```python
from build123d import *

# Parameters (mm, degrees)
F2_DEPTH    = 11.43
F0_W        = 4.9775806256
F0_H        = 21.5646
F3_DEPTH    = 3.556
F4_T1_DEPTH = 27.2262824301


# Not quite as in the source:
# - a fillet or chamfer that OpenCascade refuses, or shapes differently, is made with other operations: its cross-section is extruded or revolved along the edge and cut away or added


with BuildPart() as f2:
    # F1 (on Top) → F2 (new body)
    with BuildSketch(Plane.XY):
        with BuildLine():
            ThreePointArc((11.1534688622, 0), (0, 6.4792498177), (-11.1534688622, 0))
            Line((-11.1534688622, 0), (11.1534688622, 0))
        make_face()
    extrude(amount=F2_DEPTH)

    # F0 (on Front) → F3 (join)
    with BuildSketch(Plane.XZ):
        Rectangle(F0_W, F0_H)
    extrude(amount=F3_DEPTH)

    # F4: chamfer of 2.54 on 2 edges, made by hand

    # F4_s2 → F4_t1 (cut)
    with BuildSketch(Plane.XY.offset(-7.898141215)):
        with BuildLine():
            Line((-8.190415898, -0.0933816317), (-9.3391430842, 2.5863339915))
            Line((-9.3391430842, 2.5863339915), (-9.3759354233, 2.6213620343))
            ThreePointArc((-9.3759354233, 2.6213620343), (-10.327366328, 1.3537144774), (-11.1975980412, 0.0251645696))
            Line((-11.1975980412, 0.0251645696), (-11.1534688622, -0.0508))
            ThreePointArc((-11.1534688622, -0.0508), (-9.6719423801, -0.0508), (-8.190415898, -0.1441816317))
            Line((-8.190415898, -0.1441816317), (-8.190415898, -0.0933816317))
        make_face()
        with BuildLine():
            Line((8.190415898, -0.0933816317), (9.3391430842, 2.5863339915))
            Line((9.3391430842, 2.5863339915), (9.3759354233, 2.6213620343))
            ThreePointArc((9.3759354233, 2.6213620343), (10.327366328, 1.3537144774), (11.1975980412, 0.0251645696))
            Line((11.1975980412, 0.0251645696), (11.1534688622, -0.0508))
            ThreePointArc((11.1534688622, -0.0508), (9.6719423801, -0.0508), (8.190415898, -0.1441816317))
            Line((8.190415898, -0.1441816317), (8.190415898, -0.0933816317))
        make_face()
    extrude(amount=F4_T1_DEPTH, mode=Mode.SUBTRACT)


solid = f2.part
```
Verification items for the finished model (mm, model axes). A direction names the side the tool comes from. Coordinates: 2 decimals unless noted, no trailing zeros. Write each loop counter-clockwise with the first axis right and the second up, starting at its lowest first coordinate (ties: lowest second). Pieces come first, ordered by that corner, then holes. Notation, with made-up numbers: M 38.5,72 L 69.5,72 A18 ccw 69.5,103 Z; hole C 38,77 d10. An arc over 180 degrees is marked long. Answer as a JSON object with one key per item and string values. Group by question number.
(1) Gauge pin test, flat ends, axial feed: pin 1 (6 mm diameter, centred on x = 2.5, y = 5.5, fed in from -Z); pin 2 (9 mm diameter, centred on x = -3, z = 8, fed in from -Y); pin 3 (1.1 mm diameter, centred on y = -1, z = 5, fed in from -X); pin 4 (3 mm diameter, centred on y = -2, z = 5.5, fed in from +X). Record the tip position at first contact, or that the pin passes through.
(2) Cross-section at B-B, the plane x = 0. Record the cut outline in (y, z), and give its area (3 significant figures).
(3) Cross-section at C-C, the plane y = -0.5. Record the cut outline in (x, z), and give its area (3 significant figures).
(4) Tool access check on faces 1 (the face through (0, -2, 10.782)), 2 (the face through (2.489, -2, 0)), 3 (the face through (0, 3, 0)), 4 (the face through (-2.489, -2, 0)). Record the directions out of +Z, -Z, +X, -X, +Y, -Y that give a thin tool (end or side, any length) a straight path to the whole face; none if there is none.
(5) Cross-section at A-A, the plane z = 7.25. Record the cut outline in (x, y).
(6) Material ranges on line 1 (X direction, y = -1, z = -0.25); line 2 (Z direction, x = 3.75, y = 0.75); line 3 (Y direction, x = 1.5, z = -9.5), recorded low to high.
(7) Cross-section at D-D, the plane z = -1.5. Record the cut outline in (x, y), and give its area (3 significant figures).
Reply:
{
 "1": {"pin 1": "z = 0", "pin 2": "y = -3.56", "pin 3": "x = -2.49", "pin 4": "x = 2.49"},
 "2": {"outline": "M -3.56,-10.78 L 0,-10.78 L 0,0 L 6.48,0 L 6.48,11.43 L 0,11.43 L 0,10.78 L -3.56,10.78 Z", "area": "151 mm²"},
 "3": {"outline": "M -2.49,-10.78 L 2.49,-10.78 L 2.49,10.78 L -2.49,10.78 Z", "area": "107 mm²"},
 "4": {"face 1": "+Z, +X, -X, -Y", "face 2": "+Z, -Z, +X, -Y", "face 3": "-Z, +X, -X, +Y", "face 4": "+Z, -Z, -X, -Y"},
 "5": {"outline": "M -9.3,2.49 L -8.23,0 L -2.49,0 L -2.49,-3.56 L 2.49,-3.56 L 2.49,0 L 8.23,0 L 9.3,2.49 A12.84 ccw Z"},
 "6": {"line 1": "-2.49 to 2.49", "line 2": "0 to 11.43", "line 3": "-3.56 to 0"},
 "7": {"outline": "M -2.49,-3.56 L 2.49,-3.56 L 2.49,0 L -2.49,0 Z", "area": "17.7 mm²"}
}
